Part model, mm, in its own coordinate system. A direction names the side the tool comes from. Round coordinates to 2 decimals unless told otherwise and drop trailing zeros. Write each loop counter-clockwise with the first axis right and the second up, starting at its lowest first coordinate (ties: lowest second). Pieces come first, ordered by that corner, then holes. Notation, with made-up numbers: (87.25, 81.5) -> (96.25, 81.5) arc R22 ccw to (96.25, 88.5) -> close; hole circle Ø7 at (47.25, 7.25). An arc over 180 degrees is marked (long way). Use CSV: the item, a comma, the result in double quotes. Start each with the question number.
(1) Saw through at B-B (y = -6). Give the cut face in (x, z).
(2) Saw through at C-C (x = -0.45). Give the cut face in (y, z).
(3) Saw through at A-A (z = 0.8). Give the cut face in (x, y), plus the area to 3 significant figures.
(4) Two-plate mould, pull along X, no slides. Class faces 1 (the flat face through (0, -7, 1)), 2 (the flat face through (0.45, 2.61, 0.49)), 3 (the flat face through (-1.446, 4.972, 0.493)): released by +X, released by -X, zero draft, split by the parting line, or undercut.
(5) Probe line 1 (X direction, y = -18.5, z = 0.8); line 2 (Y direction, x = 0.85, z = 0.9); line 3 (X direction, y = 2.75, z = 0.45). List the from-to ranges inside material, lowest first. Write a range as [from, to].
(6) Which spindle directions (+Z, -Z, +X, -X, +Y, -Y) get a long thin tool onto all of the face, cutting with end or side? Do faces 4 (the flat face through (1.446, 4.972, 0.493)), 5 (the flat face through (-1.5, -7.8, 0.5)), 6 (the flat face through (-0.45, 2.61, 0.49)), 7 (the flat face through (1.5, -7.8, 0.5)). Say none if no direction does.
```python
from build123d import *

# Parameters (mm, degrees)
PAD003_DEPTH        = 1
MIRRORED005_FACE6_W = 3
MIRRORED005_FACE6_H = 1
PAD004_DEPTH        = 20


with BuildPart() as part:
    # Sketch006 → Pad003 (new body)
    with BuildSketch(Plane.XY):
        with BuildLine():
            Line((0, 0), (1.5, 0))
            Line((1.5, 0), (1.5, 4.160967))
            Line((1.5, 4.160967), (2.1, 4.160967))
            Line((2.1, 4.160967), (2.1, 4.943956))
            Line((0.810822, 5), (2.1, 4.943956))
            Line((0.098879, 0.28507), (0.810822, 5))
            ThreePointArc((0, 0.2), (0.065219, 0.224194), (0.098879, 0.28507))
            Line((0, 0), (0, 0.2))
        make_face()
    pad003 = extrude(amount=PAD003_DEPTH)

    # Mirrored005: Pad003 across Sketch006 V_Axis
    add(pad003.mirror(Plane(origin=(0, 0, 0), x_dir=(0, 0, 1), z_dir=(1, 0, 0))))

    # Mirrored005 Face6 → Pad004 (add)
    with BuildSketch(Plane(origin=(0, 0, 0.5), x_dir=(-1, 0, 0), z_dir=(0, -1, 0))):
        Rectangle(MIRRORED005_FACE6_W, MIRRORED005_FACE6_H)
    extrude(amount=PAD004_DEPTH)


solid = part.part
```
Answers:
1,outline,"(-1.5, 0) -> (1.5, 0) -> (1.5, 1) -> (-1.5, 1) -> close"
2,outline,"(-20, 0) -> (2.61, 0) -> (2.61, 1) -> (-20, 1) -> close"
3,outline,"(-2.1, 4.16) -> (-1.5, 4.16) -> (-1.5, -20) -> (1.5, -20) -> (1.5, 4.16) -> (2.1, 4.16) -> (2.1, 4.94) -> (0.81, 5) -> (0.1, 0.29) arc R0.1 cw to (0, 0.2) arc R0.1 cw to (-0.1, 0.29) -> (-0.81, 5) -> (-2.1, 4.94) -> close"
3,area,"71.6 mm²"
4,face 1,"zero draft"
4,face 2,"undercut"
4,face 3,"released by -X"
5,line 1,"x = [-1.5, 1.5]"
5,line 2,"y = [-20, 5]"
5,line 3,"x = [-1.5, -0.47], [0.47, 1.5]"
6,face 4,"+Z, -Z, +X, +Y"
6,face 5,"+Z, -Z, -X, -Y"
6,face 6,"+Z, -Z, +Y"
6,face 7,"+Z, -Z, +X, -Y"
